Design review of the part built by this model. Coordinates are the model's own, in mm. A direction names the side the tool comes from. Coordinates: 2 decimals unless noted, no trailing zeros. Loops run counter-clockwise (first coordinate to the right, second up) from the corner with the lowest first, then second, coordinate; pieces in that order, holes last.
Q1. Wall thickness on probe 1 along X at (y, z) = (7, -0.25); probe 2 along Z at (x, y) = (-7.5, 2.5); probe 3 along X at (y, z) = (34, 2.5): over which ranges is each line inside the solid? List them lowest first.
Q2. Machinability: for faces 1 (the face through (0, 37, 0)), 2 (the face through (-9.76, 19.76, -2.17)), which of the approach directions +Z, -Z, +X, -X, +Y, -Y give a long, thin tool a straight path to every point of the face, cutting with its end or side? Answer none if there is none.
Q3. Add section C-C on y = 20.5. Give the boundary of the cut face in (x, z).
Q4. For P1, Ø10, axis at y = 21.5, z = 2, coming from the +X side; P2, Ø10, axis at x = -2, y = 7.5, coming from the -Z side; P3, Ø1.5, axis at y = 32.5, z = 6.5, coming from the +X side, all flat-tipped, find the tip position at first contact; note any pin that passes through.
```python
from build123d import *

# Parameters (mm, degrees)
ESQUISSE1_R        = 13
BOSS_EXTRU_3_DEPTH = 3
CHANFREIN2_SIZE    = 3
ESQUISSE3_R        = 10
BOSS_EXTRU_4_DEPTH = 34


with BuildPart() as part:
    # Esquisse1 → Boss.-Extru.3 (new body)
    with BuildSketch(Plane(origin=(0, 0, 0), x_dir=(1, 0, 0), z_dir=(0, 1, 0))):
        with Locations(Location((0, 0, 0), (0, 0, 270))):
            Circle(ESQUISSE1_R)
    extrude(amount=BOSS_EXTRU_3_DEPTH)

    # Chanfrein2
    chanfrein2_edges = [part.edges().sort_by_distance(p)[0] for p in [
        (0, 3, -13),
    ]]
    chamfer(chanfrein2_edges, length=CHANFREIN2_SIZE - 0.0001)  # a hair under: the kernel refuses the full size

    # Esquisse3 → Boss.-Extru.4 (add)
    with BuildSketch(Plane(origin=(0, 3, 0), x_dir=(1, 0, 0), z_dir=(0, 1, 0))):
        with Locations(Location((0, 0, 0), (0, 0, 270))):
            Circle(ESQUISSE3_R)
    extrude(amount=BOSS_EXTRU_4_DEPTH)


solid = part.part
```
Entries:
1. probe 1: x = -10 to 10
1. probe 2: z = -7.35 to 7.35
1. probe 3: x = -9.68 to 9.68
2. face 1: +Z, -Z, +X, -X, +Y
2. face 2: +Y
3. outline: circle Ø20 at (0, 0)
4. P1: stops at x = 10
4. P2: stops at z = -10.37
4. P3: stops at x = 8.18
